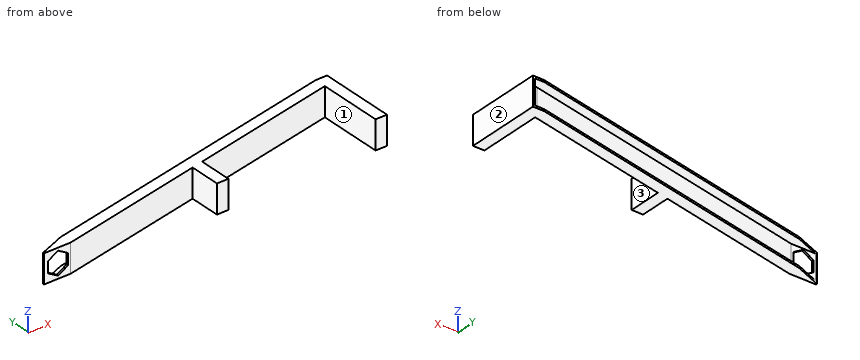
from build123d import *

# Parameters (mm, degrees)
BOSS_EXTRUDE2_DEPTH = 75
SHELL1_T            = -5
CUT_EXTRUDE2_DEPTH  = 60
CUT_EXTRUDE4_DEPTH  = 90
SKETCH12_W          = 30
SKETCH12_H          = 169.335306301
BOSS_EXTRUDE5_DEPTH = 75


with BuildPart() as part:
    # Sketch2 → Boss-Extrude2 (new body)
    with BuildSketch(Plane.XY):
        Polygon((0, 0), (70, 0), (870, 169.335306301), (900, 169.335306301), (900, 200), (870, 200), (66.859751398, 30), (0, 30), align=None)
    extrude(amount=BOSS_EXTRUDE2_DEPTH)

    # Shell1
    shell1_openings = [part.faces().sort_by_distance(p)[0] for p in [
        (33.429875699, 30, 37.5),
        (468.429875699, 115, 37.5),
        (885, 200, 37.5),
    ]]
    offset(amount=SHELL1_T, openings=shell1_openings, kind=Kind.INTERSECTION)

    # Sketch9 → Cut-Extrude2 (cut)
    with BuildSketch(Plane(origin=(0, 5, 0), x_dir=(1, 0, 0), z_dir=(0, 1, 0))):
        Polygon((37.210185308, -7.581831093), (11.229423195, -22.581831093), (11.229423195, -52.581831093), (37.210185308, -67.581831093), (63.190947422, -52.581831093), (63.190947422, -22.581831093), align=None)
    extrude(amount=-CUT_EXTRUDE2_DEPTH, mode=Mode.SUBTRACT)

    # Sketch11 → Cut-Extrude4 (cut)
    with BuildSketch(Plane.XY.offset(75)):
        Polygon((66.859751398, 30), (40.895726077, 19.305163659), (0, 3), (0, 30), align=None)
    extrude(amount=-CUT_EXTRUDE4_DEPTH, mode=Mode.SUBTRACT)

    # Sketch12 → Boss-Extrude5 (add)
    with BuildSketch(Plane.XY.offset(75)):
        with Locations((885, 84.667653151)):
            Rectangle(SKETCH12_W, SKETCH12_H)
        Polygon((453.833635791, 81.245732857), (453.833635791, 0), (483.833635791, 0), (483.833635791, 87.595806843), align=None)
    extrude(amount=-BOSS_EXTRUDE5_DEPTH)


solid = part.part
Work out the finished part from the listing and answer in its coordinate system (mm). Face numbers are marked on the shaded views. Give positions to 0.01 mm unless a question says otherwise; leave off trailing zeros. Write each loop counter-clockwise with the first axis right and the second up, starting at its lowest first coordinate (ties: lowest second). Pieces come first, ordered by that corner, then holes.
Q1. The part is cut by section C-C on y = 120. Give the vertices of the cut face in (x, z), and give its area (3 significant figures).
Answer:
outline: (492.05, 0) - (636.92, 0) - (636.92, 75) - (492.05, 75) - (492.05, 70) - (612.78, 70) - (612.78, 5) - (492.05, 5) - close; (870, 0) - (900, 0) - (900, 75) - (870, 75) - close
area: 5,270 mm2
Q2. The part is cut by section B-B on y = 46.5. Give the vertices of the cut face in (x, z).
Answer:
outline: (144.81, 0) - (289.68, 0) - (289.68, 75) - (144.81, 75) - (144.81, 70) - (265.54, 70) - (265.54, 5) - (144.81, 5) - close; (453.83, 0) - (483.83, 0) - (483.83, 75) - (453.83, 75) - close; (870, 0) - (900, 0) - (900, 75) - (870, 75) - close
Q3. The part is cut by section D-D on x = 746.5. Give the vertices of the cut face in (y, z).
Answer:
outline: (143.19, 0) - (173.86, 0) - (173.86, 5) - (148.3, 5) - (148.3, 70) - (173.86, 70) - (173.86, 75) - (143.19, 75) - close
Q4. Straight lines are drawn through the part: L1, parallel to Z at x = 738.5, y = 161; L2, parallel to Y at x = 362.5, z = 59.5; L3, parallel to Y at x = 470.5, z = 53. For each, find the intervals that lie inside material, in ascending order.
Answer:
L1: z = 0 to 5, 70 to 75
L2: y = 61.91 to 67.02
L3: y = 0 to 89.88
Q5. The part is cut by section A-A on z = 36. Give the vertices of the cut face in (x, y).
Answer:
outline: (0, 0) - (11.23, 0) - (11.23, 5) - (5.02, 5) - (0, 3) - close; (63.19, 0) - (70, 0) - (453.83, 81.25) - (453.83, 0) - (483.83, 0) - (483.83, 87.6) - (870, 169.34) - (870, 0) - (900, 0) - (900, 200) - (895, 200) - (895, 174.34) - (869.48, 174.34) - (69.48, 5) - (63.19, 5) - close
Q6. For a pull along X with two mould halves and no side action, classify the marked faces 1, 2 and 3 as released by +X, released by -X, zero draft, split by the parting line, or undercut.
Answer:
face 1: undercut
face 2: released by +X
face 3: undercut
Q7. Given pin 1 (7.5 mm diameter, centred on x = 887.5, z = 25, fed in from +Y); pin 2 (2 mm diameter, centred on x = 604, z = 41.5, fed in from -Y); pin 3 (1 mm diameter, centred on x = 151, z = 33.5, fed in from +Y), each flat-ended and moving along its own axis, determine where each tip first touches the part or whether it passes through.
Answer:
pin 1: stops at y = 174.34
pin 2: stops at y = 112.82
pin 3: stops at y = 22.36
